Geometry check sheet. Reference: the model listing, model coordinates, mm. Face numbers are marked on the shaded views. A direction names the side the tool comes from. Round coordinates to 2 decimals unless told otherwise and drop trailing zeros. Write each loop counter-clockwise with the first axis right and the second up, starting at its lowest first coordinate (ties: lowest second). Pieces come first, ordered by that corner, then holes. Notation, with made-up numbers: (35, 58) - (64, 58) arc R20 ccw to (64, 89) - close; hole circle Ø7 at (50.25, 11.25). An arc over 180 degrees is marked (long way). Return JSON: item names as keys, results as strings.
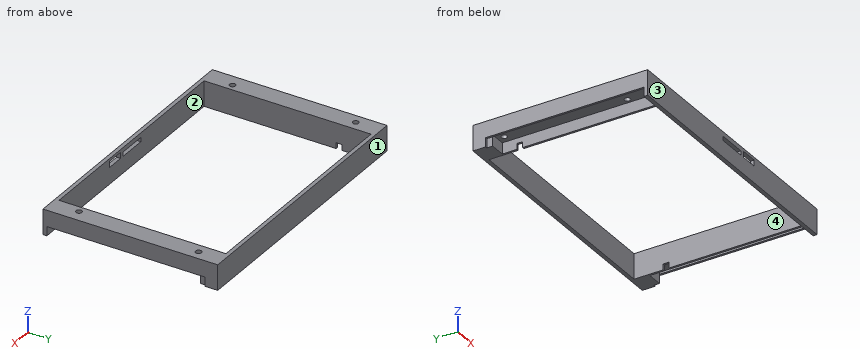
```python
from build123d import *

# Parameters (mm, degrees)
SKETCH1_W           = 140
SKETCH1_H           = 90
SKETCH1_W_2         = 120
SKETCH1_H_2         = 86
BOSS_EXTRUDE1_DEPTH = 13
SKETCH13_R          = 1.5
SKETCH13_W          = 4.8
SKETCH13_H          = 4
CUT_EXTRUDE5_DEPTH  = 5.7
SKETCH13_6_W        = 1
SKETCH13_6_H        = 5
SKETCH13_6_H_2      = 4
CUT_EXTRUDE6_DEPTH  = 4.7
SKETCH13_7_R        = 1.5
CUT_EXTRUDE7_DEPTH  = 90.528818352
SKETCH15_W          = 3
SKETCH15_H          = 3
CUT_EXTRUDE8_DEPTH  = 10
SKETCH16_W          = 1
SKETCH16_H          = 4.7
CUT_EXTRUDE9_DEPTH  = 0.5
SKETCH16_3_W        = 1
SKETCH16_3_H        = 4.7
CUT_EXTRUDE10_DEPTH = 3.5
SKETCH17_W          = 2
SKETCH17_H          = 2
CUT_EXTRUDE11_DEPTH = 1
SKETCH18_W          = 14.8
SKETCH18_H          = 2.2
SKETCH18_W_2        = 9
SKETCH18_H_2        = 3.1
CUT_EXTRUDE13_DEPTH = 2


with BuildPart() as part:
    # Sketch1 → Boss-Extrude1 (new body)
    with BuildSketch(Plane.XY):
        with Locations((1.473041333, -7.32603251)):
            Rectangle(SKETCH1_W, SKETCH1_H)
        with Locations((1.473041333, -7.32603251)):
            Rectangle(SKETCH1_W_2, SKETCH1_H_2, mode=Mode.SUBTRACT)
    extrude(amount=BOSS_EXTRUDE1_DEPTH)

    # Sketch13 → Cut-Extrude5 (cut)
    # profile 1 of 2: a face of its own
    with BuildSketch(Plane(origin=(0, 0, 0), x_dir=(-1, 0, 0), z_dir=(0, 0, -1))):
        Polygon((59.526958667, 27.67396749), (59.526958667, -50.32603251), (67.526958667, -50.32603251), (67.526958667, -45.32603251), (62.726958667, -45.32603251), (62.726958667, -41.32603251), (67.526958667, -41.32603251), (67.526958667, 27.67396749), align=None)
        with Locations((62.026958667, -37.82603251)):
            Circle(SKETCH13_R, mode=Mode.SUBTRACT)
        with Locations((63.526958667, 24.67396749)):
            Circle(SKETCH13_R, mode=Mode.SUBTRACT)
    # profile 2 of 2: a face of its own
    with BuildSketch(Plane(origin=(0, 0, 0), x_dir=(-1, 0, 0), z_dir=(0, 0, -1))):
        with Locations((65.126958667, -43.32603251)):
            Rectangle(SKETCH13_W, SKETCH13_H)
    cut_extrude5 = extrude(amount=-CUT_EXTRUDE5_DEPTH, mode=Mode.SUBTRACT)

    # Sketch13<6> → Cut-Extrude6 (cut)
    with BuildSketch(Plane(origin=(0, 0, 0), x_dir=(-1, 0, 0), z_dir=(0, 0, -1))):
        Polygon((67.526958667, 30.67396749), (67.526958667, 27.67396749), (67.526958667, -41.32603251), (68.526958667, -41.32603251), (68.526958667, 30.67396749), align=None)
        with Locations((68.026958667, -47.82603251)):
            Rectangle(SKETCH13_6_W, SKETCH13_6_H)
        with Locations((68.026958667, -43.32603251)):
            Rectangle(SKETCH13_6_W, SKETCH13_6_H_2)
    cut_extrude6 = extrude(amount=-CUT_EXTRUDE6_DEPTH, mode=Mode.SUBTRACT)

    # Sketch13<7> → Cut-Extrude7 (cut, symmetric)
    with BuildSketch(Plane(origin=(0, 0, 0), x_dir=(-1, 0, 0), z_dir=(0, 0, -1))):
        with Locations((62.026958667, -37.82603251)):
            Circle(SKETCH13_7_R)
        with Locations((63.526958667, 24.67396749)):
            Circle(SKETCH13_7_R)
    cut_extrude7 = extrude(amount=CUT_EXTRUDE7_DEPTH, both=True, mode=Mode.SUBTRACT)

    # Sketch15 → Cut-Extrude8 (cut)
    with BuildSketch(Plane.ZY.offset(-61.473041333)):
        with Locations((1.5, 19.17396749)):
            Rectangle(SKETCH15_W, SKETCH15_H)
    cut_extrude8 = extrude(amount=-CUT_EXTRUDE8_DEPTH, mode=Mode.SUBTRACT)

    # Mirror1: Cut-Extrude5, Cut-Extrude6, Cut-Extrude7, Cut-Extrude8 across plane
    add(cut_extrude5.mirror(Plane(origin=(1.473041333, 0, 0), x_dir=(0, 0, 1), z_dir=(1, 0, 0))), mode=Mode.SUBTRACT)
    add(cut_extrude6.mirror(Plane(origin=(1.473041333, 0, 0), x_dir=(0, 0, 1), z_dir=(1, 0, 0))), mode=Mode.SUBTRACT)
    add(cut_extrude7.mirror(Plane(origin=(1.473041333, 0, 0), x_dir=(0, 0, 1), z_dir=(1, 0, 0))), mode=Mode.SUBTRACT)
    add(cut_extrude8.mirror(Plane(origin=(1.473041333, 0, 0), x_dir=(0, 0, 1), z_dir=(1, 0, 0))), mode=Mode.SUBTRACT)

    # Sketch16 → Cut-Extrude9 (cut)
    with BuildSketch(Plane.XZ.offset(-27.67396749)):
        Polygon((-59.526958667, 0), (-59.526958667, 5.7), (-67.526958667, 5.7), (-67.526958667, 4.7), (-67.526958667, 0), align=None)
        with Locations((-68.026958667, 2.35)):
            Rectangle(SKETCH16_W, SKETCH16_H)
        Polygon((70.473041333, 5.7), (62.473041333, 5.7), (62.473041333, 0), (70.473041333, 0), (70.473041333, 4.7), align=None)
        with Locations((70.973041333, 2.35)):
            Rectangle(SKETCH16_W, SKETCH16_H)
    extrude(amount=-CUT_EXTRUDE9_DEPTH, mode=Mode.SUBTRACT)

    # Sketch16<3> → Cut-Extrude10 (cut)
    with BuildSketch(Plane.XZ.offset(-27.67396749)):
        with Locations((-68.026958667, 2.35)):
            Rectangle(SKETCH16_3_W, SKETCH16_3_H)
        with Locations((70.973041333, 2.35)):
            Rectangle(SKETCH16_3_W, SKETCH16_3_H)
    extrude(amount=-CUT_EXTRUDE10_DEPTH, mode=Mode.SUBTRACT)

    # Sketch17 → Cut-Extrude11 (cut)
    with BuildSketch(Plane(origin=(0, -50.32603251, 0), x_dir=(1, 0, 0), z_dir=(0, 1, 0))):
        with Locations((-64.026958667, -4.7)):
            Rectangle(SKETCH17_W, SKETCH17_H)
        with Locations((66.973041333, -4.7)):
            Rectangle(SKETCH17_W, SKETCH17_H)
    extrude(amount=-CUT_EXTRUDE11_DEPTH, mode=Mode.SUBTRACT)

    # Sketch18 → Cut-Extrude13 (cut)
    with BuildSketch(Plane(origin=(0, -52.32603251, 0), x_dir=(1, 0, 0), z_dir=(0, 1, 0))):
        with Locations((1.073041333, -9.6)):
            Rectangle(SKETCH18_W, SKETCH18_H)
        with Locations((14.973041333, -10.05)):
            Rectangle(SKETCH18_W_2, SKETCH18_H_2)
    extrude(amount=CUT_EXTRUDE13_DEPTH, mode=Mode.SUBTRACT)


solid = part.part
```
(1) Section check B-B, the plane x = 52. Enter the section's corners in (y, z).
Response values:
{"outline": "(-52.33, 0) - (-50.33, 0) - (-50.33, 13) - (-52.33, 13) - close; (35.67, 0) - (37.67, 0) - (37.67, 13) - (35.67, 13) - close"}
(2) Gauge pin test, flat ends, axial feed: pin 1 (2.5 mm diameter, centred on x = 67.5, y = -25, fed in from -Z); pin 2 (1.7 mm diameter, centred on y = 3.5, z = 2, fed in from +X). Record the tip position at first contact, or that the pin passes through.
Response values:
{"pin 1": "stops at z = 5.7", "pin 2": "stops at x = 62.47"}
(3) Section check A-A, the plane x = 16. Enter the section's corners in (y, z), plus the area to 3 significant figures.
Response values:
{"outline": "(-52.33, 0) - (-50.33, 0) - (-50.33, 8.5) - (-52.33, 8.5) - close; (-52.33, 11.6) - (-50.33, 11.6) - (-50.33, 13) - (-52.33, 13) - close; (35.67, 0) - (37.67, 0) - (37.67, 13) - (35.67, 13) - close", "area": "45.8 mm^2"}
(4) Section check C-C, the plane y = -41. Enter the section's corners in (x, z), plus the area to 3 significant figures.
Response values:
{"outline": "(-68.53, 4.7) - (-67.53, 4.7) - (-67.53, 5.7) - (-59.53, 5.7) - (-59.53, 0) - (-58.53, 0) - (-58.53, 13) - (-68.53, 13) - close; (61.47, 0) - (62.47, 0) - (62.47, 5.7) - (70.47, 5.7) - (70.47, 4.7) - (71.47, 4.7) - (71.47, 13) - (61.47, 13) - close", "area": "159 mm^2"}
(5) Access from +Z, -Z, +X, -X, +Y, -Y to the whole of each face (thin tool, end or side, straight path). Record for the marked faces 1 and 2.
Response values:
{"face 1": "+Z, -Z, +X, -X, +Y", "face 2": "+Z, -Z"}
(6) Release check for a two-part mould opening along X. For the marked faces 3 and 4 record: pulls with the +X half, pulls with the -X half, needs draft (parallel to the pull), parting line crosses it, or undercut.
Response values:
{"face 3": "needs draft", "face 4": "undercut"}
(7) Material ranges on line 1 along X through (y, z) = (-18, 5.5); line 2 along X through (y, z) = (-45, 2); line 3 along X through (y, z) = (24.5, 8), recorded low to high. Write a range as [from, to].
Response values:
{"line 1": "x = [-68.53, -67.53], [-59.53, -58.53], [61.47, 62.47], [70.47, 71.47]", "line 2": "x = [-59.53, -58.53], [61.47, 62.47]", "line 3": "x = [-68.53, -65.02], [-62.04, -58.53], [61.47, 64.98], [67.96, 71.47]"}
